Build history of the part. All positions in model axes, mm. A direction names the side the tool comes from. Give positions to 0.01 mm unless a question says otherwise; leave off trailing zeros. Order: outer loops, then holes, each group sorted by start corner. A loop starts at its lowest first (then second) coordinate and runs counter-clockwise, first axis right, second up. Notation, with made-up numbers: (63.5, 14.5) - (120.5, 14.5) arc R16 cw to (120.5, 40.5) - close; hole circle Ø9 at (31.5, -11.5). An arc over 180 degrees is marked (long way). Answer in a Markdown table with one row per item.
```python
from build123d import *

# Parameters (mm, degrees)
BOSS_EXTRUDE1_DEPTH = 1.524
CUT_EXTRUDE1_DEPTH  = 1.524


with BuildPart() as part:
    # Sketch1 → Boss-Extrude1 (new body)
    with BuildSketch(Plane.XY):
        with BuildLine():
            Line((57.290824473, 228.108297044), (353.711488573, 186.321991739))
            ThreePointArc((353.711488573, 186.321991739), (354.075780486, 186.801693195), (354.433282196, 187.286476253))
            ThreePointArc((354.433282196, 187.286476253), (367.282944414, 188.133579217), (379.736207542, 191.411938565))
            ThreePointArc((379.736207542, 191.411938565), (342.378628376, 201.501430101), (311.755483248, 225.157497886))
            ThreePointArc((311.755483248, 225.157497886), (300.682282637, 235.370307227), (300.562470929, 250.433603398))
            ThreePointArc((300.562470929, 250.433603398), (321.044455039, 268.037495843), (343.59946469, 282.892806069))
            ThreePointArc((343.59946469, 282.892806069), (377.376618301, 298.266191923), (413.38768552, 307.235034456))
            ThreePointArc((413.38768552, 307.235034456), (393.078041438, 309.22946311), (373.338877641, 304.050196657))
            ThreePointArc((373.338877641, 304.050196657), (345.164765747, 299.513120241), (316.730515739, 297.09256867))
            ThreePointArc((316.730515739, 297.09256867), (300.377514826, 294.830345717), (283.869742792, 294.652149172))
            ThreePointArc((283.869742792, 294.652149172), (264.837645669, 295.417547796), (246.095409129, 292.02120779))
            ThreePointArc((246.095409129, 292.02120779), (215.671555063, 284.944519585), (184.616227681, 281.589366329))
            ThreePointArc((184.616227681, 281.589366329), (167.005302639, 283.674185668), (150.340503018, 289.738475081))
            ThreePointArc((150.340503018, 289.738475081), (157.435124743, 294.404562686), (165.406340408, 297.331293248))
            ThreePointArc((165.406340408, 297.331293248), (159.650281584, 297.625042258), (153.959513951, 296.711989461))
            ThreePointArc((153.959513951, 296.711989461), (144.425837897, 293.107350234), (135.76973662, 287.726243123))
            ThreePointArc((135.76973662, 287.726243123), (131.283660572, 283.993726612), (125.519570472, 283.081683228))
            ThreePointArc((125.519570472, 283.081683228), (117.575446144, 283.528434685), (109.74705726, 282.10540072))
            ThreePointArc((109.74705726, 282.10540072), (105.901175076, 281.967449489), (104.441699592, 285.528316185))
            ThreePointArc((104.441699592, 285.528316185), (106.645115294, 290.563839268), (109.921107262, 294.977387738))
            ThreePointArc((109.921107262, 294.977387738), (105.298186283, 293.444448732), (101.575381834, 290.304062227))
            ThreePointArc((101.575381834, 290.304062227), (89.522712553, 279.763084543), (75.355674106, 272.301578731))
            ThreePointArc((75.355674106, 272.301578731), (75.025286429, 278.530980407), (77.97930542, 284.025375103))
            ThreePointArc((77.97930542, 284.025375103), (70.672937053, 278.271974974), (68.631929607, 269.198997493))
            ThreePointArc((68.631929607, 269.198997493), (60.712120021, 259.329966949), (51.319192238, 250.850930717))
            ThreePointArc((51.319192238, 250.850930717), (47.204267049, 247.59528857), (42.038095614, 246.677417222))
            ThreePointArc((42.038095614, 246.677417222), (27.881645016, 252.981360845), (16.64661192, 263.65463729))
            ThreePointArc((16.64661192, 263.65463729), (14.473805053, 264.820038124), (13.469532472, 262.568219888))
            ThreePointArc((13.469532472, 262.568219888), (21.739819765, 249.170959745), (34.989718338, 240.66658328))
            ThreePointArc((34.989718338, 240.66658328), (45.889493734, 233.942107147), (57.290824473, 228.108297044))
        make_face()
        with BuildLine():
            ThreePointArc((328.489226954, 199.182421433), (244.252401976, 213.020971981), (159.578269796, 223.867146564))
            ThreePointArc((159.578269796, 223.867146564), (232.039463881, 246.03834442), (301.131135651, 277.159519764))
            ThreePointArc((301.131135651, 277.159519764), (291.304602068, 264.568913579), (283.869742792, 250.433603398))
            ThreePointArc((283.869742792, 250.433603398), (298.334085197, 217.977776055), (328.489226954, 199.182421433))
        make_face(mode=Mode.SUBTRACT)
        with BuildLine():
            ThreePointArc((73.889360105, 231.521400998), (65.868365727, 237.228895624), (68.631929607, 246.677417222))
            ThreePointArc((68.631929607, 246.677417222), (70.855224439, 249.097244695), (73.19077168, 251.408915949))
            ThreePointArc((73.19077168, 251.408915949), (71.867025962, 241.406389626), (73.889360105, 231.521400998))
        make_face(mode=Mode.SUBTRACT)
        with BuildLine():
            ThreePointArc((116.551068066, 270.179316334), (122.101400858, 269.279382121), (127.7241229, 269.312131715))
            ThreePointArc((127.7241229, 269.312131715), (131.669689581, 246.96106507), (140.187225602, 225.923259654))
            ThreePointArc((140.187225602, 225.923259654), (118.722956961, 228.014416663), (97.240833112, 229.913395557))
            ThreePointArc((97.240833112, 229.913395557), (95.566690644, 249.574533087), (102.786152544, 267.938695246))
            ThreePointArc((102.786152544, 267.938695246), (109.612083308, 269.406270814), (116.551068066, 270.179316334))
        make_face(mode=Mode.SUBTRACT)
        with BuildLine():
            ThreePointArc((147.854387632, 278.340365744), (191.622365865, 273.02026195), (235.390344097, 278.340365744))
            ThreePointArc((235.390344097, 278.340365744), (259.286439501, 284.470493189), (283.869742792, 282.405780779))
            ThreePointArc((283.869742792, 282.405780779), (290.901656942, 281.917548628), (297.936216355, 282.366058505))
            ThreePointArc((297.936216355, 282.366058505), (225.245012107, 250.01614522), (148.884216081, 227.665375775))
            ThreePointArc((148.884216081, 227.665375775), (142.212285393, 251.073648633), (144.166314335, 275.335628523))
            ThreePointArc((144.166314335, 275.335628523), (146.063284577, 276.773025404), (147.854387632, 278.340365744))
        make_face(mode=Mode.SUBTRACT)
        with BuildLine():
            ThreePointArc((92.963126534, 264.492689611), (88.906900231, 247.537272471), (91.873275106, 230.357640278))
            ThreePointArc((91.873275106, 230.357640278), (86.092526476, 230.822576823), (80.310675632, 231.273599578))
            ThreePointArc((80.310675632, 231.273599578), (76.354412107, 241.989032993), (75.355674106, 253.367743674))
            ThreePointArc((75.355674106, 253.367743674), (83.738923989, 259.595704551), (92.963126534, 264.492689611))
        make_face(mode=Mode.SUBTRACT)
    extrude(amount=BOSS_EXTRUDE1_DEPTH)

    # Sketch2 → Cut-Extrude1 (cut)
    with BuildSketch(Plane(origin=(0, 0, 0), x_dir=(-1, 0, 0), z_dir=(0, 0, -1))):
        Polygon((-293.228442315, 248.191486466), (-292.963264261, 246.690734455), (-301.831560839, 245.123734967), (-302.096738893, 246.624486978), align=None)
        Polygon((-210.010989789, 277.610431446), (-208.536964433, 277.452860551), (-207.725093618, 285.047652502), (-209.384282149, 285.202159423), align=None)
        Polygon((-61.191894588, 250.827806426), (-60.009228178, 249.866621656), (-54.939782062, 256.104198263), (-56.208453293, 256.959560494), align=None)
    extrude(amount=-CUT_EXTRUDE1_DEPTH, mode=Mode.SUBTRACT)


solid = part.part
```
1. Cut at A-A on x = 349. Write the cut outline in (y, z), and give its area (3 significant figures).
Check result:
| item | result |
|---|---|
| outline | (186.99, 0) - (198.51, 0) - (198.51, 1.52) - (186.99, 1.52) - close; (285.87, 0) - (300, 0) - (300, 1.52) - (285.87, 1.52) - close |
| area | 39.1 mm² |
2. Probe line 1 (Y direction, x = 161, z = 0.65); line 2 (Y direction, x = 200, z = 1.45); line 3 (Y direction, x = 234, z = 1.45). List the from-to ranges inside material, lowest first.
Check result:
| item | result |
|---|---|
| line 1 | y = 213.49 to 223.71, 224.21 to 230.48, 275.6 to 285.36, 295.97 to 297.66 |
| line 2 | y = 207.99 to 219.07, 235 to 241.39, 273.21 to 282.78 |
| line 3 | y = 203.2 to 214.5, 246.78 to 253.31, 278 to 288.74 |
3. Cut at D-D on z = 0.85. Count the separate pieces of the cut face and the enclosed holes in it, and give its area (3 significant figures).
Check result:
| item | result |
|---|---|
| separate pieces | 1 |
| enclosed holes | 5 |
| area | 11,600 mm² |
4. Which spindle directions (+Z, -Z, +X, -X, +Y, -Y) get a long thin tool onto all of the face, cutting with end or side? Do faces 5 (the face through (258.94, 284.44, 0.75)), 6 (the face through (376.9, 298.1, 0.8)), 7 (the face through (212, 244, 1.524)). Say none if no direction does.
Check result:
| item | result |
|---|---|
| face 5 | +Z, -Z |
| face 6 | +Z, -Z, +X |
| face 7 | +Z, +X, -X, +Y, -Y |
5. Two-plate mould, pull along Y, no slides. Class faces 1 (the face through (28.063, 252.861, 0.751)), 2 (the face through (167.247, 283.617, 0.751)), 3 (the face through (203.426, 207.508, 0.751)), 4 (the face through (131.58, 247.27, 0.75)): +Y half, -Y half, draft (parallel to the pull), parting line (faces both ways), or undercut.
Check result:
| item | result |
|---|---|
| face 1 | +Y half |
| face 2 | undercut |
| face 3 | -Y half |
| face 4 | undercut |
6. Cut at C-C on x = 173. Write the cut outline in (y, z), and give its area (3 significant figures).
Check result:
| item | result |
|---|---|
| outline | (211.8, 0) - (222.35, 0) - (222.35, 1.52) - (211.8, 1.52) - close; (227.23, 0) - (233.53, 0) - (233.53, 1.52) - (227.23, 1.52) - close; (273.97, 0) - (282.5, 0) - (282.5, 1.52) - (273.97, 1.52) - close |
| area | 38.7 mm² |
